Design review of the part built by this model. Coordinates are the model's own, in mm. A direction names the side the tool comes from. Give positions to 0.01 mm unless a question says otherwise; leave off trailing zeros. Write each loop counter-clockwise with the first axis right and the second up, starting at its lowest first coordinate (ties: lowest second). Pieces come first, ordered by that corner, then holes. Notation, with made-up numbers: (47.25, 49) -> (96.25, 49) arc R21 ccw to (96.25, 83) -> close; hole circle Ø4 at (-2.5, -9.5). An arc over 180 degrees is marked (long way). Answer as a JSON object with one key per item and string values.
```python
from build123d import *

# Parameters (mm, degrees)
F0_W     = 70
F0_H     = 75
F1_DEPTH = 100
F2_W     = 40
F2_H     = 25
F3_DEPTH = 100.001
F4_W     = 40
F4_H     = 25
F5_DEPTH = 75.001
F6_R     = 25
F7_DEPTH = 75.001
F8_W     = 25
F8_H     = 20
F9_DEPTH = 15


with BuildPart() as f1:
    # F0 (on Front) → F1 (new body)
    with BuildSketch(Plane.XZ):
        with Locations((35, 37.5)):
            Rectangle(F0_W, F0_H)
    extrude(amount=-F1_DEPTH)

    # F2 (on face) → F3 (cut, through all)
    with BuildSketch(Plane.XZ):
        with Locations((50, 12.5)):
            Rectangle(F2_W, F2_H)
    extrude(amount=-F3_DEPTH, mode=Mode.SUBTRACT)

    # F4 (on face) → F5 (cut, through all)
    with BuildSketch(Plane.XY.offset(75)):
        with Locations((50, 87.5)):
            Rectangle(F4_W, F4_H)
    extrude(amount=-F5_DEPTH, mode=Mode.SUBTRACT)

    # F6 (on face) → F7 (cut, through all)
    with BuildSketch(Plane.XY.offset(75)):
        with Locations((40, 40)):
            Circle(F6_R)
    extrude(amount=-F7_DEPTH, mode=Mode.SUBTRACT)

    # F8 (on face) → F9 (cut)
    with BuildSketch(Plane.XY.offset(75)):
        with Locations((17.5, 85)):
            Rectangle(F8_W, F8_H)
    extrude(amount=-F9_DEPTH, mode=Mode.SUBTRACT)


solid = f1.part
```
(1) We need section D-D, the plane x = 25. State the section outline as (y, z) points, then the cut area to 3 significant figures.
Here are the results:
{"outline": "(0, 0) -> (20, 0) -> (20, 75) -> (0, 75) -> close; (60, 0) -> (100, 0) -> (100, 75) -> (95, 75) -> (95, 60) -> (75, 60) -> (75, 75) -> (60, 75) -> close", "area": "4,200 mm²"}
(2) Clearance check with flat-ended pins moving along their axes: pin 1 (6 mm diameter, centred on x = 16.5, y = 86.5, fed in from +Z); pin 2 (19 mm diameter, centred on y = 5, z = 7, fed in from +X); pin 3 (12 mm diameter, centred on x = 51.5, y = 23.5, fed in from -Z). State where each tip first meets the part, or that it passes through.
Here are the results:
{"pin 1": "stops at z = 60", "pin 2": "stops at x = 30", "pin 3": "stops at z = 25"}
(3) We need section C-C, the plane y = 40. State the section outline as (x, z) points, then the cut area to 4 significant figures.
Here are the results:
{"outline": "(0, 0) -> (15, 0) -> (15, 75) -> (0, 75) -> close; (65, 25) -> (70, 25) -> (70, 75) -> (65, 75) -> close", "area": "1,375 mm²"}
(4) The part is to be moulded in two halves that separate along Y. For faces 4 (the flat face through (15, 100, 38)), 5 (the flat face through (5, 85, 68)), 6 (the flat face through (44, 75, 56)), 7 (the flat face through (30, 8, 12)), say which applies: +Y half, -Y half, draft (parallel to the pull), parting line (faces both ways), or undercut.
Here are the results:
{"face 4": "+Y half", "face 5": "undercut", "face 6": "undercut", "face 7": "draft"}
(5) For faces 1 (the flat face through (63, 29, 25)), 2 (the flat face through (17, 85, 60)), 3 (the flat face through (15, 49, 0)), list the 3-axis set-ups (+Z, -Z, +X, -X, +Y, -Y) from which the entire face can be reached by the end or side of a thin tool; tool diameter is ignored.
Here are the results:
{"face 1": "-Z, +X, +Y, -Y", "face 2": "+Z, +X", "face 3": "-Z, +X, -X, +Y, -Y"}
(6) We need section A-A, the plane x = 40. State the section outline as (y, z) points, then the cut area to 3 significant figures.
Here are the results:
{"outline": "(0, 25) -> (15, 25) -> (15, 75) -> (0, 75) -> close; (65, 25) -> (75, 25) -> (75, 75) -> (65, 75) -> close", "area": "1,250 mm²"}
(7) For line 1 along Y through (x, z) = (40, 60); line 2 along X through (y, z) = (40, 46); line 3 along X through (y, z) = (76.5, 54), list the stretches that pass through material, from the lowest coordinate up.
Here are the results:
{"line 1": "y = 0 to 15, 65 to 75", "line 2": "x = 0 to 15, 65 to 70", "line 3": "x = 0 to 30"}
(8) We need section B-B, the plane z = 28. State the section outline as (x, y) points, then the cut area to 3 significant figures.
Here are the results:
{"outline": "(0, 0) -> (70, 0) -> (70, 75) -> (30, 75) -> (30, 100) -> (0, 100) -> close; hole circle Ø50 at (40, 40)", "area": "4,040 mm²"}
